Read the model definition and answer for the solid it produces. Units are mm, in the model's axes. A direction names the side the tool comes from. Coordinates: 2 decimals unless noted, no trailing zeros. Loops run counter-clockwise (first coordinate to the right, second up) from the corner with the lowest first, then second, coordinate; pieces in that order, holes last.
from build123d import *

# Parameters (mm, degrees)
ESQUISSE1_W             = 140
ESQUISSE1_H             = 30
ESQUISSE1_R             = 11
ESQUISSE1_R_2           = 6
EXTRUSION1_DEPTH        = 8
ESQUISSE2_W             = 140
ESQUISSE2_H             = 50
BOSS_EXTRU_1_DEPTH      = 4
ESQUISSE3_R             = 3
ENL_V_MAT_EXTRU_1_DEPTH = 13
ESQUISSE4_R             = 11
ENL_V_MAT_EXTRU_2_DEPTH = 2
ESQUISSE5_W             = 100
ESQUISSE5_H             = 20
BOSS_EXTRU_2_DEPTH      = 8
ESQUISSE6_R             = 3
ENL_V_MAT_EXTRU_3_DEPTH = 8
ESQUISSE8_R             = 6
ENL_V_MAT_EXTRU_4_DEPTH = 2
ESQUISSE9_R             = 11
ESQUISSE9_R_2           = 4.5
BOSS_EXTRU_3_DEPTH      = 3
ESQUISSE10_R            = 3
ENL_V_MAT_EXTRU_5_DEPTH = 13
CONG_1_R                = 2
CONG_2_R                = 2


with BuildPart() as part:
    # Esquisse1 → Extrusion1 (new body)
    with BuildSketch(Plane.XY):
        with Locations((9.95634141, -28.081325038)):
            Rectangle(ESQUISSE1_W, ESQUISSE1_H)
        with Locations((9.95634141, -28.081325038)):
            Circle(ESQUISSE1_R, mode=Mode.SUBTRACT)
        with Locations((-40.04365859, -28.081325038)):
            Circle(ESQUISSE1_R_2, mode=Mode.SUBTRACT)
        with Locations((59.95634141, -28.081325038)):
            Circle(ESQUISSE1_R_2, mode=Mode.SUBTRACT)
    extrude(amount=EXTRUSION1_DEPTH)

    # Esquisse2 → Boss.-Extru.1 (add)
    with BuildSketch(Plane(origin=(0, 0, 0), x_dir=(-1, 0, 0), z_dir=(0, 0, -1))):
        with Locations((-9.95634141, -38.081325038)):
            Rectangle(ESQUISSE2_W, ESQUISSE2_H)
    extrude(amount=BOSS_EXTRU_1_DEPTH)

    # Esquisse3 → Enlèv. mat.-Extru.1 (cut, through all)
    with BuildSketch(Plane(origin=(0, 0, -4), x_dir=(-1, 0, 0), z_dir=(0, 0, -1))):
        with Locations((-69.95634141, -53.081325038)):
            Circle(ESQUISSE3_R)
        with Locations((50.04365859, -53.081325038)):
            Circle(ESQUISSE3_R)
    extrude(amount=-ENL_V_MAT_EXTRU_1_DEPTH, mode=Mode.SUBTRACT)

    # Esquisse4 → Enlèv. mat.-Extru.2 (cut)
    with BuildSketch(Plane.XY):
        with Locations((9.95634141, -28.081325038)):
            Circle(ESQUISSE4_R)
    extrude(amount=-ENL_V_MAT_EXTRU_2_DEPTH, mode=Mode.SUBTRACT)

    # Esquisse5 → Boss.-Extru.2 (add)
    with BuildSketch(Plane.XY):
        with Locations((9.95634141, -53.081325038)):
            Rectangle(ESQUISSE5_W, ESQUISSE5_H)
    extrude(amount=BOSS_EXTRU_2_DEPTH)

    # Esquisse6 → Enlèv. mat.-Extru.3 (cut)
    with BuildSketch(Plane.XY.offset(8)):
        with Locations((22.95634141, -58.081325038)):
            Circle(ESQUISSE6_R)
        with Locations((-3.04365859, -58.081325038)):
            Circle(ESQUISSE6_R)
    extrude(amount=-ENL_V_MAT_EXTRU_3_DEPTH, mode=Mode.SUBTRACT)

    # Esquisse8 → Enlèv. mat.-Extru.4 (cut)
    with BuildSketch(Plane.XY):
        with Locations((-40.04365859, -28.081325038)):
            Circle(ESQUISSE8_R)
        with Locations((59.95634141, -28.081325038)):
            Circle(ESQUISSE8_R)
    extrude(amount=-ENL_V_MAT_EXTRU_4_DEPTH, mode=Mode.SUBTRACT)

    # Esquisse9 → Boss.-Extru.3 (add)
    with BuildSketch(Plane.XY.offset(-2)):
        with Locations((9.95634141, -28.081325038)):
            Circle(ESQUISSE9_R)
        with Locations((9.95634141, -28.081325038)):
            Circle(ESQUISSE9_R_2, mode=Mode.SUBTRACT)
    extrude(amount=BOSS_EXTRU_3_DEPTH)

    # Esquisse10 → Enlèv. mat.-Extru.5 (cut, through all)
    with BuildSketch(Plane.XY.offset(8)):
        with Locations((9.95634141, -58.081325038)):
            Circle(ESQUISSE10_R)
    extrude(amount=-ENL_V_MAT_EXTRU_5_DEPTH, mode=Mode.SUBTRACT)

    # Congé1
    cong_1_edges = [part.edges().sort_by_distance(p)[0] for p in [
        (-40.04365859, -43.081325038, 4),
    ]]
    fillet(cong_1_edges, radius=CONG_1_R)

    # Congé2
    cong_2_edges = [part.edges().sort_by_distance(p)[0] for p in [
        (59.95634141, -43.081325038, 4),
    ]]
    fillet(cong_2_edges, radius=CONG_2_R)


solid = part.part
Q1. A cutting plane is placed at A-A (y = -37.5). Give the vertices of the cut face in (x, z).
Findings below:
outline: (-60.04, -4) - (79.96, -4) - (79.96, 8) - (15.64, 8) - (15.64, 1) - (4.27, 1) - (4.27, 8) - (-60.04, 8) - close
Q2. Flat-ended cylindrical pins translate along their axes: pin 1 Ø3 at (x, y) = (-4, -57.5) entering from +Z; pin 2 Ø4 at (x, z) = (-50.5, 4.5) entering from -Y; pin 3 Ø7 at (x, y) = (9, -28.5) entering from +Z; pin 4 Ø3.5 at (x, y) = (9.96, -58.08) entering from +Z. Find the tip coordinate at first contact, or state that the pin passes through.
Findings below:
pin 1: stops at z = 0
pin 2: stops at y = -43.08
pin 3: stops at z = 1
pin 4: passes through
Q3. Determine the mould class of faces 5 (the face through (-60.044, -33, 1)), 6 (the face through (-51, -43.081, 4)), 7 (the face through (79.956, -33, 1)), 8 (the face through (-3, -58, 0)) for opening direction X: +X half, -X half, draft (parallel to the pull), parting line (faces both ways), or undercut.
Findings below:
face 5: -X half
face 6: draft
face 7: +X half
face 8: undercut
Q4. Straight lines are drawn through the part: probe 1 along X at (y, z) = (-27.5, 6.5); probe 2 along X at (y, z) = (-30.5, 7.25); probe 3 along Z at (x, y) = (3.5, -21). For each, find the intervals that lie inside material, in ascending order.
Findings below:
probe 1: x = -60.04 to -46.02, -34.07 to -1.03, 20.94 to 53.98, 65.93 to 79.96
probe 2: x = -60.04 to -45.53, -34.55 to -0.77, 20.69 to 54.47, 65.45 to 79.96
probe 3: z = -4 to 1
Q5. A cutting plane is placed at B-B (z = 3). Give the vertices of the cut face in (x, y), then the cut area to 3 significant figures.
Findings below:
outline: (-60.04, -43.08) - (-42.04, -43.08) arc R2 cw to (-40.04, -45.08) - (-40.04, -63.08) - (59.96, -63.08) - (59.96, -45.08) arc R2 cw to (61.96, -43.08) - (79.96, -43.08) - (79.96, -13.08) - (-60.04, -13.08) - close; hole circle Ø12 at (-40.04, -28.08); hole circle Ø6 at (-3.04, -58.08); hole circle Ø22 at (9.96, -28.08); hole circle Ø6 at (9.96, -58.08); hole circle Ø6 at (22.96, -58.08); hole circle Ø12 at (59.96, -28.08)
area: 5,510 mm2
Q6. Which of the six approach directions +Z, -Z, +X, -X, +Y, -Y give full straight-line access (tool end or side, diameter ignored) to faces 1 (the face through (72.3, -50.7, 0)), 2 (the face through (-47.7, -50.7, 0)), 3 (the face through (11, -38, -4)), 4 (the face through (7.57, -38.82, 4.45))?
Findings below:
face 1: +Z, +X, -Y
face 2: +Z, -X, -Y
face 3: -Z, +X, -X, +Y, -Y
face 4: +Z
Q7. A cutting plane is placed at C-C (x = 4). Give the vertices of the cut face in (y, z).
Findings below:
outline: (-63.08, -4) - (-13.08, -4) - (-13.08, 8) - (-18.83, 8) - (-18.83, 1) - (-37.33, 1) - (-37.33, 8) - (-63.08, 8) - close
